Design review of the part built by this model. Coordinates are the model's own, in mm. Face numbers are marked on the shaded views. A direction names the side the tool comes from. Coordinates: 2 decimals unless noted, no trailing zeros. Loops run counter-clockwise (first coordinate to the right, second up) from the corner with the lowest first, then second, coordinate; pieces in that order, holes last. Notation, with made-up numbers: (39, 42.25) -> (87, 42.25) arc R25 ccw to (87, 74.25) -> close; hole circle Ø5 at (-12, -37.5). An arc over 180 degrees is marked (long way). Use one line per item in the form item = value. Start each with the question number.
1. Machinability: for the marked faces 4, 5 and 6, which of the approach directions +Z, -Z, +X, -X, +Y, -Y give a long, thin tool a straight path to every point of the face, cutting with its end or side? Answer none if there is none.
2. Wall thickness on line 1 (X direction, y = 58, z = -20.5); line 2 (Y direction, x = -32, z = -31); line 3 (Z direction, x = -0.5, y = 9.5) (3 decimals): over which ranges is each line inside the solid? List them lowest first. Write a range as from..to.
3. For pin 1 (1 mm diameter, centred on x = -4, z = -33.5, fed in from -Y), flat-tipped, find the tip position at first contact; note if it passes through.
4. The part is to be moulded in two halves that separate along X. For the marked faces 1, 2 and 3, say which applies: released by +X, released by -X, zero draft, split by the parting line, or undercut.
5. Consider section C-C (y = 48.5). State the section outline as (x, z) points, then the cut area to 3 significant figures.
6. Consider section B-B (x = 33). State the section outline as (y, z) points.
7. Consider section A-A (z = -7). State the section outline as (x, y) points.
8. Consider section D-D (z = -20). State the section outline as (x, y) points.
from build123d import *

# Parameters (mm, degrees)
SKETCH1_R           = 25
BOSS_EXTRUDE1_DEPTH = 10
SKETCH2_W           = 100
SKETCH2_H           = 100
BOSS_EXTRUDE2_DEPTH = 50
CUT_EXTRUDE1_DEPTH  = 127.885775404
SKETCH7_W           = 20
SKETCH7_H           = 75
CUT_EXTRUDE3_DEPTH  = 30


with BuildPart() as part:
    # Sketch1 → Boss-Extrude1 (new body)
    with BuildSketch(Plane(origin=(0, 0, 0), x_dir=(1, 0, 0), z_dir=(0, 1, 0))):
        with Locations(Location((0, 0, 0), (0, 0, 270))):
            Circle(SKETCH1_R)
    extrude(amount=BOSS_EXTRUDE1_DEPTH)

    # Sketch2 → Boss-Extrude2 (add)
    with BuildSketch(Plane(origin=(0, 10, 0), x_dir=(1, 0, 0), z_dir=(0, 1, 0))):
        Rectangle(SKETCH2_W, SKETCH2_H)
    extrude(amount=BOSS_EXTRUDE2_DEPTH)

    # Sketch4 → Cut-Extrude1 (cut, through all)
    with BuildSketch(Plane.ZY.offset(50)):
        Polygon((50, 30.318847412), (7.085498034, 60), (50, 60), align=None)
    extrude(amount=-CUT_EXTRUDE1_DEPTH, mode=Mode.SUBTRACT)

    # Sketch7 → Cut-Extrude3 (cut)
    with BuildSketch(Plane(origin=(0, 60, 0), x_dir=(1, 0, 0), z_dir=(0, 1, 0))):
        with Locations((0, -12.5)):
            Rectangle(SKETCH7_W, SKETCH7_H)
    extrude(amount=-CUT_EXTRUDE3_DEPTH, mode=Mode.SUBTRACT)


solid = part.part
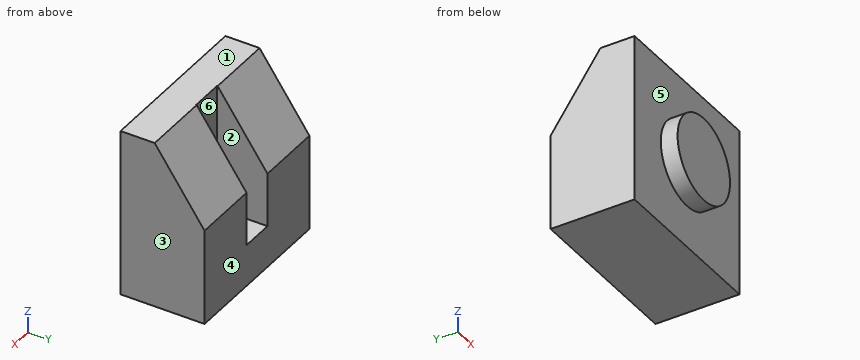
Geometry check:
q1.face_4 = +Z, -Z, +X, -X, +Y
q1.face_5 = -Y
q1.face_6 = +Z, +Y
q2.line_1 = -50..-10, 10..50
q2.line_2 = 10..60
q2.line_3 = -24.995..24.995
q3.pin_1 = 10
q4.face_1 = zero draft
q4.face_2 = undercut
q4.face_3 = released by +X
q5.outline = (-50, -50) -> (50, -50) -> (50, 23.71) -> (10, 23.71) -> (10, -25) -> (-10, -25) -> (-10, 23.71) -> (-50, 23.71) -> close
q5.area = 6,400 mm²
q6.outline = (10, -50) -> (60, -50) -> (60, 7.09) -> (30.32, 50) -> (10, 50) -> close
q7.outline = (-50, 10) -> (-24, 10) -> (-24, 0) -> (24, 0) -> (24, 10) -> (50, 10) -> (50, 60) -> (10, 60) -> (10, 30) -> (-10, 30) -> (-10, 60) -> (-50, 60) -> close
q8.outline = (-50, 10) -> (-15, 10) -> (-15, 0) -> (15, 0) -> (15, 10) -> (50, 10) -> (50, 60) -> (10, 60) -> (10, 30) -> (-10, 30) -> (-10, 60) -> (-50, 60) -> close
